For this review, take the finished solid that the model builds, in its own axes (mm). A direction names the side the tool comes from. Round coordinates to 2 decimals unless told otherwise and drop trailing zeros. Order: outer loops, then holes, each group sorted by start corner. A loop starts at its lowest first (then second) coordinate and runs counter-clockwise, first axis right, second up. Notation, with made-up numbers: (26.25, -12) -> (56.25, -12) arc R33 ccw to (56.25, 20) -> close; hole circle Ø11 at (89, 81). An arc over 180 degrees is marked (long way). Use a Markdown table: item, result. Add a question column.
1) Clearance check with flat-ended pins moving along their axes: P1, Ø5, axis at x = -291.5, z = 5, coming from the -Y side (3 decimals); P2, Ø3, axis at x = -292, z = 5, coming from the +Y side (3 decimals); P3, Ø9.5, axis at y = -116.5, z = 9, coming from the -X side (3 decimals). State where each tip first meets the part, or that it passes through.
2) Draft analysis for pull direction X (two halves, no side actions). For faces 1 (the face through (295.275, -1, 9)), 2 (the face through (107.741, 95.252, 9.658)), 3 (the face through (-195, 123.825, 10)), state which applies: pulls with the +X half, pulls with the -X half, needs draft (parallel to the pull), parting line crosses it, or undercut.
3) Consider section C-C (x = 14.5). State the section outline as (y, z) points (3 decimals), plus the area to 3 significant figures.
4) Consider section B-B (x = 107.95). State the section outline as (y, z) points.
5) Consider section A-A (z = 12.25). State the section outline as (x, y) points (3 decimals).
6) Machinability: for faces 4 (the face through (-269.875, -114, 10)), 5 (the face through (269.875, 114, 10)), 6 (the face through (-1, -104.775, 9)), 7 (the face through (193, 123.825, 10)), 8 (the face through (117.475, 114, 10)), which of the approach directions +Z, -Z, +X, -X, +Y, -Y give a long, thin tool a straight path to every point of the face, cutting with its end or side? Answer none if there is none.
7) Wall thickness on line 1 along X through (y, z) = (-106.5, 14.5) (3 decimals); line 2 along X through (y, z) = (-101, 9.5) (3 decimals); line 3 along Y through (x, z) = (-82, 5) (3 decimals): over which ranges is each line inside the solid? List them lowest first. Write a range as [from, to].
```python
from build123d import *

# Parameters (mm, degrees)
F1_W     = 590.55
F1_H     = 209.55
F2_DEPTH = 19.05
F3_W     = 152.4
F3_H     = 247.65
F4_DEPTH = 19.05
F6_DEPTH = 25.4


# Not quite as in the source:
# - a variable given as a bare number and used for a length is read in inches; the dataset says mm whatever the document's units were


with BuildPart() as f2:
    # F1 (on Top) → F2 (new body)
    with BuildSketch(Plane.XY):
        Rectangle(F1_W, F1_H)
    extrude(amount=F2_DEPTH)

    # F3 (on face) → F4 (join)
    with BuildSketch(Plane.XY.offset(19.05)):
        with Locations((-193.675, 0)):
            Rectangle(F3_W, F3_H)
        with Locations((193.675, 0)):
            Rectangle(F3_W, F3_H)
    extrude(amount=-F4_DEPTH)

    # F5 (on face) → F6 (cut)
    with BuildSketch(Plane.XY.offset(19.05)):
        with BuildLine():
            Line((-98.425, 104.775), (-117.475, 104.775))
            ThreePointArc((-117.475, 104.775), (-107.95, 95.25), (-98.425, 104.775))
        make_face()
        with BuildLine():
            ThreePointArc((-98.425, 104.775), (-107.95, 114.3), (-117.475, 104.775))
            Line((-117.475, 104.775), (-98.425, 104.775))
        make_face()
        with BuildLine():
            Line((-117.475, -104.775), (-98.425, -104.775))
            ThreePointArc((-98.425, -104.775), (-107.95, -95.25), (-117.475, -104.775))
        make_face()
        with BuildLine():
            Line((98.425, -104.775), (117.475, -104.775))
            ThreePointArc((117.475, -104.775), (107.95, -95.25), (98.425, -104.775))
        make_face()
        with BuildLine():
            Line((117.475, 104.775), (98.425, 104.775))
            ThreePointArc((98.425, 104.775), (107.95, 95.25), (117.475, 104.775))
        make_face()
        with BuildLine():
            Line((288.925, 104.775), (269.875, 104.775))
            ThreePointArc((269.875, 104.775), (279.4, 95.25), (288.925, 104.775))
        make_face()
        with BuildLine():
            Line((269.875, -104.775), (288.925, -104.775))
            ThreePointArc((288.925, -104.775), (279.4, -95.25), (269.875, -104.775))
        make_face()
        with BuildLine():
            Line((-288.925, -104.775), (-269.875, -104.775))
            ThreePointArc((-269.875, -104.775), (-279.4, -95.25), (-288.925, -104.775))
        make_face()
        with BuildLine():
            Line((-269.875, 104.775), (-288.925, 104.775))
            ThreePointArc((-288.925, 104.775), (-279.4, 95.25), (-269.875, 104.775))
        make_face()
    extrude(amount=-F6_DEPTH, mode=Mode.SUBTRACT)


solid = f2.part
```
Results list:
| question | item | result |
|---|---|---|
| 1 | P1 | y = -104.775 |
| 1 | P2 | y = 104.775 |
| 1 | P3 | x = -269.875 |
| 2 | face 1 | pulls with the +X half |
| 2 | face 2 | undercut |
| 2 | face 3 | needs draft |
| 3 | outline | (-104.775, 0) -> (104.775, 0) -> (104.775, 19.05) -> (-104.775, 19.05) -> close |
| 3 | area | 3,990 mm2 |
| 4 | outline | (-95.25, 0) -> (95.25, 0) -> (95.25, 19.05) -> (-95.25, 19.05) -> close |
| 5 | outline | (-295.275, -104.775) -> (-288.925, -104.775) arc R9.525 cw to (-269.875, -104.775) -> (-269.875, -123.825) -> (-117.475, -123.825) -> (-117.475, -104.775) arc R9.525 cw to (-98.425, -104.775) -> (98.425, -104.775) arc R9.525 cw to (117.475, -104.775) -> (117.475, -123.825) -> (269.875, -123.825) -> (269.875, -104.775) arc R9.525 cw to (288.925, -104.775) -> (295.275, -104.775) -> (295.275, 104.775) -> (288.925, 104.775) arc R9.525 cw to (269.875, 104.775) -> (269.875, 123.825) -> (117.475, 123.825) -> (117.475, 104.775) arc R9.525 cw to (98.425, 104.775) -> (-98.425, 104.775) arc R9.525 cw to (-117.475, 104.775) -> (-117.475, 123.825) -> (-269.875, 123.825) -> (-269.875, 104.775) arc R9.525 cw to (-288.925, 104.775) -> (-295.275, 104.775) -> close |
| 6 | face 4 | +Z, -Z, -X, -Y |
| 6 | face 5 | +Z, -Z, +X, +Y |
| 6 | face 6 | +Z, -Z, -Y |
| 6 | face 7 | +Z, -Z, +X, -X, +Y |
| 6 | face 8 | +Z, -Z, +Y |
| 7 | line 1 | [-269.875, -117.475], [117.475, 269.875] |
| 7 | line 2 | [-295.275, -288.145], [-270.655, -116.695], [-99.205, 99.205], [116.695, 270.655], [288.145, 295.275] |
| 7 | line 3 | [-104.775, 104.775] |
